Part model, mm, in its own coordinate system. Face numbers are marked on the shaded views. A direction names the side the tool comes from. Give positions to 0.01 mm unless a question says otherwise; leave off trailing zeros. Order: outer loops, then holes, each group sorted by start corner. A loop starts at its lowest first (then second) coordinate and runs counter-clockwise, first axis right, second up. Notation, with made-up numbers: (63, -13) - (72, -13) arc R18 ccw to (72, -2) - close; hole circle Ø10 at (-20.5, -29.75). An arc over 180 degrees is marked (long way). One line per item, written item: value.
```python
from build123d import *

# Parameters (mm, degrees)
EXTRUDE_1_DEPTH     = 4
SKETCH_1_3_R        = 2.5
CUT_EXTRUDE_1_DEPTH = 5
SKETCH_1_4_W        = 52.5
SKETCH_1_4_H        = 21
EXTRUDE_2_DEPTH     = 12.2


with BuildPart() as part:
    # Sketch 1 → Extrude 1 (new body)
    with BuildSketch(Plane(origin=(0, 0, 0), x_dir=(1, 0, 0), z_dir=(0, 1, 0))):
        with BuildLine():
            Line((-65.1, 49.6), (0, 49.6))
            ThreePointArc((0, 49.6), (5.303300859, 47.403300859), (7.5, 42.1))
            Line((7.5, 42.1), (7.5, 0))
            ThreePointArc((7.5, 0), (5.303300859, -5.303300859), (0, -7.5))
            Line((0, -7.5), (-65.1, -7.5))
            ThreePointArc((-65.1, -7.5), (-70.403300859, -5.303300859), (-72.6, 0))
            Line((-72.6, 0), (-72.6, 42.1))
            ThreePointArc((-72.6, 42.1), (-70.403300859, 47.403300859), (-65.1, 49.6))
        make_face()
    extrude(amount=EXTRUDE_1_DEPTH)

    # Sketch 1_3 → Cut-Extrude 1 (cut)
    with BuildSketch(Plane(origin=(0, 0, 0), x_dir=(1, 0, 0), z_dir=(0, 1, 0))):
        with Locations(Location((-65.1, 42.1, 0), (0, 0, 270))):
            Circle(SKETCH_1_3_R)
        with Locations(Location((0, 42.1, 0), (0, 0, 90))):
            Circle(SKETCH_1_3_R)
        with Locations(Location((0, 0, 0), (0, 0, 270))):
            Circle(SKETCH_1_3_R)
        with Locations(Location((-65.1, 0, 0), (0, 0, 90))):
            Circle(SKETCH_1_3_R)
    extrude(amount=CUT_EXTRUDE_1_DEPTH, mode=Mode.SUBTRACT)

    # Sketch 1_4 → Extrude 2 (add)
    with BuildSketch(Plane(origin=(0, 0, 0), x_dir=(1, 0, 0), z_dir=(0, 1, 0))):
        with BuildLine():
            Line((-6.204635364, 37.05), (-58.895364636, 37.05))
            ThreePointArc((-58.895364636, 37.05), (-59.779658065, 36.125557625), (-60.8, 35.35389001))
            Line((-60.8, 35.35389001), (-60.8, 12.05))
            Line((-60.8, 12.05), (-4.3, 12.05))
            Line((-4.3, 12.05), (-4.3, 35.35389001))
            ThreePointArc((-4.3, 35.35389001), (-5.320341935, 36.125557625), (-6.204635364, 37.05))
        make_face()
        with Locations((-32.55, 24.55)):
            Rectangle(SKETCH_1_4_W, SKETCH_1_4_H, mode=Mode.SUBTRACT)
    extrude(amount=EXTRUDE_2_DEPTH)


solid = part.part
```
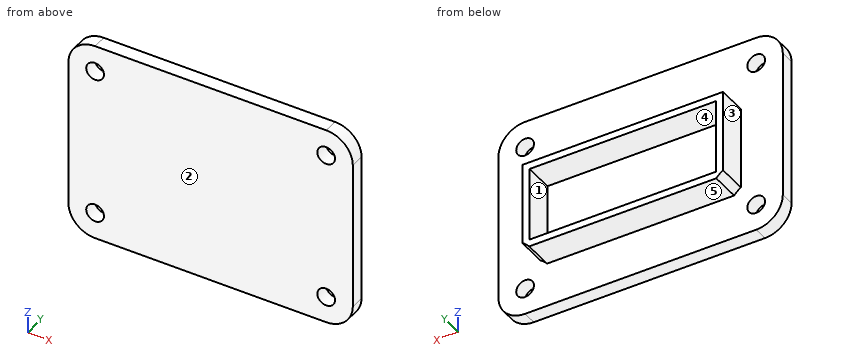
1) Which spindle directions (+Z, -Z, +X, -X, +Y, -Y) get a long thin tool onto all of the face, cutting with end or side? Do the marked faces 4 and 5. Say none if no direction does.
Outcome:
face 4: +Y
face 5: -Z, +X, -X, +Y
2) Cut at A-A, the plane y = 7.5. Give the cut face in (x, z).
Outcome:
outline: (-60.8, -35.35) arc R8 cw to (-58.9, -37.05) - (-6.2, -37.05) arc R8 cw to (-4.3, -35.35) - (-4.3, -12.05) - (-60.8, -12.05) - close; hole (-58.8, -35.05) - (-6.3, -35.05) - (-6.3, -14.05) - (-58.8, -14.05) - close
3) Cut at D-D, the plane x = -11. Give the cut face in (y, z), then the cut area to 3 significant figures.
Outcome:
outline: (0, -49.6) - (4, -49.6) - (4, -37.05) - (12.2, -37.05) - (12.2, -35.05) - (4, -35.05) - (4, -14.05) - (12.2, -14.05) - (12.2, -12.05) - (4, -12.05) - (4, 7.5) - (0, 7.5) - close
area: 261 mm^2
4) Mould opens along X. For the marked faces 1, 2 and 3 say: released by +X, released by -X, zero draft, split by the parting line, or undercut.
Outcome:
face 1: undercut
face 2: zero draft
face 3: released by -X
5) Cut at C-C, the plane y = 1. Give the cut face in (x, z).
Outcome:
outline: (-72.6, -42.1) arc R7.5 ccw to (-65.1, -49.6) - (0, -49.6) arc R7.5 ccw to (7.5, -42.1) - (7.5, 0) arc R7.5 ccw to (0, 7.5) - (-65.1, 7.5) arc R7.5 ccw to (-72.6, 0) - close; hole circle Ø5 at (-65.1, -42.1); hole circle Ø5 at (-65.1, 0); hole circle Ø5 at (0, -42.1); hole circle Ø5 at (0, 0)
6) Pin check, flat tips, straight feed: pin 1 (2.5 mm diameter, centred on x = -20.5, y = 9.5, fed in from -Z); pin 2 (17 mm diameter, centred on x = -27.5, z = -35, fed in from +Y); pin 3 (1.5 mm diameter, centred on y = 8.5, z = -32, fed in from -X); pin 4 (6 mm diameter, centred on x = -3, y = 9, fed in from +Z). Stop position of each tip, or through.
Outcome:
pin 1: stops at z = -37.05
pin 2: stops at y = 12.2
pin 3: stops at x = -60.8
pin 4: stops at z = -12.05
7) Cut at B-B, the plane z = -18.5. Give the cut face in (x, y), then the cut area to 3 significant figures.
Outcome:
outline: (-72.6, 0) - (7.5, 0) - (7.5, 4) - (-4.3, 4) - (-4.3, 12.2) - (-6.3, 12.2) - (-6.3, 4) - (-58.8, 4) - (-58.8, 12.2) - (-60.8, 12.2) - (-60.8, 4) - (-72.6, 4) - close
area: 353 mm^2
8) Drill centre lines: line 1 along Z through (x, y) = (-65.1, 1); line 2 along X through (y, z) = (1.55, -42.1); line 3 along X through (y, z) = (9.5, -24.5). Where is each one in solid material? Low to high. Write a range as from..to.
Outcome:
line 1: z = -49.6..-44.6, -39.6..-2.5, 2.5..7.5
line 2: x = -72.6..-67.6, -62.6..-2.5, 2.5..7.5
line 3: x = -60.8..-58.8, -6.3..-4.3
